```python
from build123d import *

# Parameters (mm, degrees)
DODANIE_WYCI_GNI_CIE1_DEPTH = 5.2
SZKIC6_W                    = 49.271239353
SZKIC6_H                    = 120
WYTNIJ_WYCI_GNI_CIE1_DEPTH  = 78
WYTNIJ_WYCI_GNI_CIE2_DEPTH  = 5.6
SZKIC9_R                    = 2.424871131
SZKIC9_R_2                  = 1.2
DODANIE_WYCI_GNI_CIE3_DEPTH = 3.8
SZKIC10_W                   = 50
SZKIC10_H                   = 39.9
WYTNIJ_WYCI_GNI_CIE4_DEPTH  = 24


with BuildPart() as part:
    # Szkic2 → Dodanie-wyci_gni_cie1 (new body)
    with BuildSketch(Plane.XY):
        Polygon((18.542832418, 83.245366469), (18.542832418, 43.345366469), (-51.457167582, 43.345366469), (-51.457167582, -76.654633531), (18.542832418, -76.654633531), (18.542832418, -116.554633531), (-81.357167582, -116.554633531), (-81.357167582, 83.245366469), align=None)
    extrude(amount=DODANIE_WYCI_GNI_CIE1_DEPTH)

    # Szkic3 → Wyci_gni_cie po profilach3 section 0
    with BuildSketch(Plane.XY.offset(11.5)):
        with BuildLine():
            Line((-41.457167582, -76.654633531), (18.542832418, -76.654633531))
            Line((18.542832418, -76.654633531), (18.542832418, 83.245366469))
            Line((18.542832418, 83.245366469), (-41.457167582, 83.245366469))
            Line((-41.457167582, 83.245366469), (-41.457167582, -76.654633531))
        make_face()
    # Szkic5 → Wyci_gni_cie po profilach3 section 1
    with BuildSketch(Plane.XY.offset(5.2)):
        with BuildLine():
            Line((-81.357167582, 83.245366469), (18.542832418, 83.245366469))
            Line((18.542832418, 83.245366469), (18.542832418, -116.554633531))
            Line((18.542832418, -116.554633531), (-81.357167582, -116.554633531))
            Line((-81.357167582, -116.554633531), (-81.357167582, 83.245366469))
        make_face()
    loft()

    # Szkic6 → Wytnij-wyci_gni_cie1 (cut)
    with BuildSketch(Plane(origin=(-51.457167582, 0, 0), x_dir=(0, 0, -1), z_dir=(1, 0, 0))):
        with Locations((-24.635619677, -16.654633531)):
            Rectangle(SZKIC6_W, SZKIC6_H)
    extrude(amount=WYTNIJ_WYCI_GNI_CIE1_DEPTH, mode=Mode.SUBTRACT)

    # Szkic7 → Wytnij-wyci_gni_cie2 (cut)
    with BuildSketch(Plane(origin=(-51.457167582, 0, 0), x_dir=(0, 0, -1), z_dir=(1, 0, 0))):
        Polygon((-5.12, -34.1297624), (-7.22, -35.342197966), (-7.22, -37.767069096), (-5.12, -38.979504662), (-3.02, -37.767069096), (-3.02, -35.342197966), align=None)
        Polygon((-5.12, 5.6702376), (-7.22, 4.457802034), (-7.22, 2.032930904), (-5.12, 0.820495338), (-3.02, 2.032930904), (-3.02, 4.457802034), align=None)
    extrude(amount=-WYTNIJ_WYCI_GNI_CIE2_DEPTH, mode=Mode.SUBTRACT)

    # Szkic9 → Dodanie-wyci_gni_cie3 (add)
    # profile 1 of 2: a face of its own
    with BuildSketch(Plane(origin=(-51.457167582, 0, 0), x_dir=(0, 0, -1), z_dir=(1, 0, 0))):
        with Locations((-5.12, 3.245366469)):
            Circle(SZKIC9_R)
        with Locations(Location((-5.12, 3.245366469, 0), (0, 0, 90))):
            Circle(SZKIC9_R_2, mode=Mode.SUBTRACT)
    # profile 2 of 2: a face of its own
    with BuildSketch(Plane(origin=(-51.457167582, 0, 0), x_dir=(0, 0, -1), z_dir=(1, 0, 0))):
        with Locations((-5.12, -36.554633531)):
            Circle(SZKIC9_R)
        with Locations(Location((-5.12, -36.554633531, 0), (0, 0, 90))):
            Circle(SZKIC9_R_2, mode=Mode.SUBTRACT)
    extrude(amount=-DODANIE_WYCI_GNI_CIE3_DEPTH)

    # Szkic10 → Wytnij-wyci_gni_cie4 (cut)
    with BuildSketch(Plane.XY.offset(11.5)):
        with Locations((-6.457167582, 63.295366469)):
            Rectangle(SZKIC10_W, SZKIC10_H)
    extrude(amount=-WYTNIJ_WYCI_GNI_CIE4_DEPTH, mode=Mode.SUBTRACT)


solid = part.part
```
Design review of the part built by this model. Coordinates are the model's own, in mm. A direction names the side the tool comes from. Coordinates: 2 decimals unless noted, no trailing zeros.
Q1. For pin 1 (1.4 mm diameter, centred on x = -56, y = -36.5, fed in from +Z); pin 2 (3 mm diameter, centred on y = 3.25, z = 5.12, fed in from +X); pin 3 (0.5 mm diameter, centred on x = -56, y = 3, fed in from +Z), all flat-tipped, find the tip position at first contact; note any pin that passes through.
Reported:
pin 1: stops at z = 9.31
pin 2: stops at x = -51.46
pin 3: stops at z = 9.24
Q2. Tool access review of faces 4 (the face through (-36, 63, 11.5)), 5 (the face through (-42, 43.345, 6)), 6 (the face through (-31.457, 63, 6)), 7 (the face through (-57.057, -37, 5)): name each direction out of +Z, -Z, +X, -X, +Y, -Y from which nothing blocks a thin tool from reaching the whole face with its end or side.
Reported:
face 4: +Z, +X, -X, +Y, -Y
face 5: +Z, -Z, +X
face 6: +Z, -Z, +X, +Y
face 7: none
Q3. To check wall thickness, follow line 1 (Y direction, x = -39, z = 4.5); line 2 (X direction, y = 8, z = 0.5); line 3 (Y direction, x = -7, z = 1.25). State the ranges of each line that lie inside material, in increasing order.
Reported:
line 1: y = -116.55 to -76.65, 43.35 to 83.25
line 2: x = -81.36 to -51.46
line 3: y = -116.55 to -76.65
Q4. The part is to be moulded in two halves that separate along Y. For faces 1 (the face through (-31, -116.555, 3)), 2 (the face through (-81.357, -18, 3)), 3 (the face through (-55.257, -38, 6)), say which applies: +Y half, -Y half, draft (parallel to the pull), parting line (faces both ways), or undercut.
Reported:
face 1: -Y half
face 2: draft
face 3: undercut
